Job drawing, mm, ordinate dimensions from the low corner. One solid piece. A direction names the side the tool comes from. Give positions to 0.01 mm unless a question says otherwise; leave off trailing zeros. Loops run counter-clockwise (first coordinate to the right, second up) from the corner with the lowest first, then second, coordinate; pieces in that order, holes last. Notation, with made-up numbers: M -8.5,-30 L 1.5,-30 A31 ccw 1.5,3 Z; hole C 38.25,-16.75 d4. An arc over 180 degrees is marked long. Put each result on its own line as item: value.
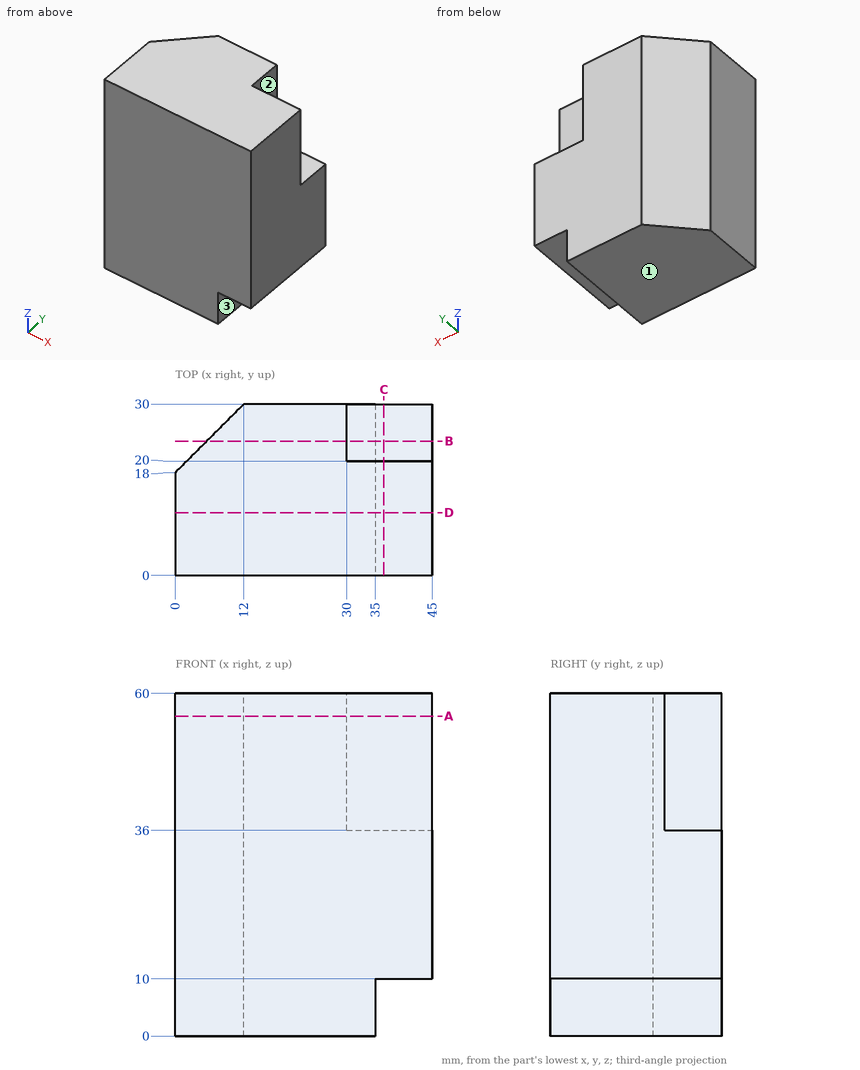
Q1. Drop flat-ended pins along their axis: pin 1 Ø3 at (y, z) = (27.5, 50) entering from +X; pin 2 Ø3 at (x, y) = (38, 15.5) entering from -Z; pin 3 Ø5 at (x, y) = (40, 27.5) entering from +Z. Give the stop position or say it passes through.
Here are the results:
pin 1: x = 30
pin 2: z = 10
pin 3: z = 36
Q2. Slice it at D-D (y = 11). List the corners of the cut face in (x, z), and give its area (3 significant figures).
Here are the results:
outline: M 0,0 L 35,0 L 35,10 L 45,10 L 45,60 L 0,60 Z
area: 2,600 mm²
Q3. Slice it at A-A (z = 56). List the corners of the cut face in (x, y).
Here are the results:
outline: M 0,0 L 45,0 L 45,20 L 30,20 L 30,30 L 12,30 L 0,18 Z
Q4. Probe line 1 (X direction, y = 28, z = 13); line 2 (Z direction, x = 39, y = 6.5); line 3 (Z direction, x = 39, y = 25). List the from-to ranges inside material, lowest first. Write a range as from..to.
Here are the results:
line 1: 10..45
line 2: 10..60
line 3: 10..36
Q5. Slice it at C-C (x = 36.5). List the corners of the cut face in (y, z).
Here are the results:
outline: M 0,10 L 30,10 L 30,36 L 20,36 L 20,60 L 0,60 Z
Q6. Tool access for the marked faces 1, 2 and 3: list every direction of +Z, -Z, +X, -X, +Y, -Y with a clear straight run to the whole face (end or side of a thin tool).
Here are the results:
face 1: -Z, +X, -X, +Y, -Y
face 2: +Z, +X, +Y
face 3: -Z, +X, +Y, -Y
Q7. Slice it at B-B (y = 23.5). List the corners of the cut face in (x, z).
Here are the results:
outline: M 5.5,0 L 35,0 L 35,10 L 45,10 L 45,36 L 30,36 L 30,60 L 5.5,60 Z
